Design review of the part built by this model. Coordinates are the model's own, in mm. A direction names the side the tool comes from. Coordinates: 2 decimals unless noted, no trailing zeros. Order: outer loops, then holes, each group sorted by start corner. A loop starts at its lowest first (then second) coordinate and runs counter-clockwise, first axis right, second up. Notation, with made-up numbers: (70, 2) - (88, 2) arc R13 cw to (88, 12) - close; hole circle Ø5 at (-11.75, 40). An arc over 180 degrees is marked (long way). Write item = value, one per line. Start each with the question number.
```python
from build123d import *

# Parameters (mm, degrees)
SKETCH_1_R      = 1
EXTRUDE_1_DEPTH = 1.5


with BuildPart() as part:
    # 草图1 → 凸台-拉伸1 (new body)
    with BuildSketch(Plane.XY):
        with BuildLine():
            Line((10.83152947, -1.623168698), (-30.649174333, -59.245657467))
            ThreePointArc((-30.649174333, -59.245657467), (-31.464927374, -62.837478083), (-33.476977186, -59.752306464))
            Line((-33.476977186, -59.752306464), (-1.116519701, -11.659332323))
            ThreePointArc((-1.116519701, -11.659332323), (-1.912938139, -9.416332563), (0, -8))
            Line((0, -8), (0, -2))
            ThreePointArc((0, -2), (-1.414213562, 1.414213562), (2, 0))
            Line((2, 0), (10, 0))
            ThreePointArc((10, 0), (13.780019812, 0.911882377), (10.83152947, -1.623168698))
        make_face()
        with Locations((-31.817644863, -60.868826165)):
            Circle(SKETCH_1_R, mode=Mode.SUBTRACT)
        Circle(SKETCH_1_R, mode=Mode.SUBTRACT)
        with Locations((12, 0)):
            Circle(SKETCH_1_R, mode=Mode.SUBTRACT)
        with Locations((0, -10)):
            Circle(SKETCH_1_R, mode=Mode.SUBTRACT)
    extrude(amount=EXTRUDE_1_DEPTH)


solid = part.part
```
Item 1: For faces 1 (the flat face through (0, -5, 1)), 2 (the flat face through (-8, -23, 1.5)), 3 (the flat face through (6, 0, 1)), list the 3-axis set-ups (+Z, -Z, +X, -X, +Y, -Y) from which the entire face can be reached by the end or side of a thin tool; tool diameter is ignored.
Item 2: Add section D-D on x = -22.5. Give the boundary of the cut face in (y, z), plus the area to 3 significant figures.
Item 3: Add section C-C on z = 0.5. Give the boundary of the cut face in (x, y), plus the area to 3 significant figures.
Item 4: Add section B-B on y = -10. Give the boundary of the cut face in (x, z), plus the area to 3 significant figures.
Item 5: For line 1 (Y direction, x = 12, z = 0.4); line 2 (X direction, y = -23, z = 0.8); line 3 (X direction, y = -26.5, z = 1.45), list the stretches that pass through material, from the lowest coordinate up.
Item 6: Add section A-A on x = 12. Give the boundary of the cut face in (y, z), plus the area to 3 significant figures.
Item 7: Mouldability with a two-part tool opening along X and no side actions: class faces 4 (the cylindrical face through (-31.401, -62.825, 0.74)), 5 (the cylindrical face through (-1.923, -9.451, 0.74)), 6 (the cylindrical face through (13.745, 0.978, 0.74)), 7 (the flat face through (-8, -23, 0)) as +X half, -X half, draft (parallel to the pull), parting line (faces both ways), or undercut.
Worked out:
q1.face_1 = +Z, -Z, -X
q1.face_2 = +Z, +X, -X, +Y, -Y
q1.face_3 = +Z, -Z, +Y
q2.outline = (-47.93, 0) - (-43.44, 0) - (-43.44, 1.5) - (-47.93, 1.5) - close
q2.area = 6.73 mm2
q3.outline = (-33.48, -59.75) arc R2 ccw (long way) to (-30.65, -59.25) - (10.83, -1.62) arc R2 ccw (long way) to (10, 0) - (2, 0) arc R2 ccw (long way) to (0, -2) - (0, -8) arc R2 ccw to (-1.12, -11.66) - close; hole circle Ø2 at (-31.82, -60.87); hole circle Ø2 at (0, -10); hole circle Ø2 at (0, 0); hole circle Ø2 at (12, 0)
q3.area = 288 mm2
q4.outline = (-2, 0) - (-1, 0) - (-1, 1.5) - (-2, 1.5) - close; (1, 0) - (4.8, 0) - (4.8, 1.5) - (1, 1.5) - close
q4.area = 7.20 mm2
q5.line_1 = -2 to -1, 1 to 2
q5.line_2 = -8.75 to -4.56
q5.line_3 = -11.1 to -7.08
q6.outline = (-2, 0) - (-1, 0) - (-1, 1.5) - (-2, 1.5) - close; (1, 0) - (2, 0) - (2, 1.5) - (1, 1.5) - close
q6.area = 3.00 mm2
q7.face_4 = parting line
q7.face_5 = -X half
q7.face_6 = undercut
q7.face_7 = draft
